from build123d import *

# Parameters (mm, degrees)
F0_R       = 50
F1_DEPTH   = 200
F2_R       = 30
F3_DEPTH   = 150
F1_FACE1_R = 50
F4_R       = 10
F5_DEPTH   = 50
F6_R       = 10
F7_DEPTH   = 150
F8_W       = 25
F8_H       = 25
F8_R       = 10
F9_DEPTH   = 50


# Not quite as in the source:
# - a fillet or chamfer that OpenCascade refuses, or shapes differently, is made with other operations: its cross-section is extruded or revolved along the edge and cut away or added


with BuildPart() as f1:
    # F0 (on Top) → F1 (new body)
    with BuildSketch(Plane.XY):
        Circle(F0_R)
    extrude(amount=F1_DEPTH)

    # F2 (on face) → F3 (cut)
    with BuildSketch(Plane.XY.offset(200)):
        Circle(F2_R)
    extrude(amount=-F3_DEPTH, mode=Mode.SUBTRACT)

    # F1_face1 (on face) + F4 (on face) → F5 (join)
    with BuildSketch(Plane(origin=(0, 0, 0), x_dir=(1, 0, 0), z_dir=(0, 0, -1))):
        Circle(F1_FACE1_R)
    with BuildSketch(Plane(origin=(0, 0, 0), x_dir=(1, 0, 0), z_dir=(0, 0, -1))):
        Circle(F4_R)
    extrude(amount=F5_DEPTH)

    # F6 (on face) → F7 (cut)
    with BuildSketch(Plane(origin=(0, 0, -50), x_dir=(1, 0, 0), z_dir=(0, 0, -1))):
        Circle(F6_R)
    extrude(amount=-F7_DEPTH, mode=Mode.SUBTRACT)

    # F8 (on face) → F9 (join)
    with BuildSketch(Plane.XY.offset(50)):
        Rectangle(F8_W, F8_H)
        Circle(F8_R, mode=Mode.SUBTRACT)
    extrude(amount=F9_DEPTH)

    # F10: chamfer of 15 on 1 edges, made by hand

    # F10_s1 → F10_t2 (revolve)
    with BuildSketch(Plane.XZ):
        Polygon((30, 65), (15, 50), (30, 50), align=None)
    revolve(axis=Axis((0, 0, 50), (0, 0, 1)))


solid = f1.part
Source: CAD feature listing. Evaluate the final solid. Frame: model axes, mm. A direction names the side the tool comes from. Give positions to 0.01 mm unless a question says otherwise; leave off trailing zeros. Write each loop counter-clockwise with the first axis right and the second up, starting at its lowest first coordinate (ties: lowest second). Pieces come first, ordered by that corner, then holes. Notation, with made-up numbers: (40, 64) -> (48, 64) arc R13 cw to (48, 83) -> close; hole circle Ø1 at (81.5, 78.5). An arc over 180 degrees is marked (long way). Return JSON: item names as keys, results as strings. Group by question number.
1. Section A-A, the plane z = 90.5. Output: boundary loops of the cut face in (x, y).
2. Section D-D, the plane z = 38. Output: boundary loops of the cut face in (x, y).
3. Section B-B, the plane x = 0. Output: boundary loops of the cut face in (y, z), then the cut area to 3 significant figures.
4. Pin query (flat end, axial travel): pin 1 Ø12 at (y, z) = (-20, 123.5) entering from +X; pin 2 Ø0.8 at (x, y) = (13.5, -3.5) entering from +Z; pin 3 Ø12.5 at (x, z) = (0.5, 70) entering from -Y. Return the tip coordinate at first contact, or that it passes through.
5. Mould query, pull axis Y, two halves, no side actions, for faces 3 (the face through (47.69, -15.02, 76.75)), 4 (the face through (-0.7, 10.4, -50)), 5 (the face through (-12.5, 0, 75)). Classes: +Y half, -Y half, draft (parallel to the pull), parting line (faces both ways), or undercut.
6. Material intervals for line 1 (X direction, y = 0, z = 29); line 2 (Y direction, x = 0, z = 129.5), sorted ascending. Write a range as from..to.
7. Access query for faces 1 (the face through (-2.17, -9.76, 23.95)), 2 (the face through (-9, 6, 100)). Directions: +Z, -Z, +X, -X, +Y, -Y. A direction counts if a zero-diameter tool reaches every point of the face in a straight line with its end or side. Return the directions, or none.
Determined:
{
 "1": {"outline": "circle Ø100 at (0, 0); (-12.5, -12.5) -> (12.5, -12.5) -> (12.5, 12.5) -> (-12.5, 12.5) -> close; hole circle Ø60 at (0, 0); hole circle Ø20 at (0, 0)"},
 "2": {"outline": "circle Ø100 at (0, 0); hole circle Ø20 at (0, 0)"},
 "3": {"outline": "(-50, -50) -> (-10, -50) -> (-10, 100) -> (-12.5, 100) -> (-12.5, 50) -> (-15, 50) -> (-30, 65) -> (-30, 200) -> (-50, 200) -> close; (10, -50) -> (50, -50) -> (50, 200) -> (30, 200) -> (30, 65) -> (15, 50) -> (12.5, 50) -> (12.5, 100) -> (10, 100) -> close", "area": "14,500 mm2"},
 "4": {"pin 1": "stops at x = 48", "pin 2": "stops at z = 50", "pin 3": "stops at y = -50"},
 "5": {"face 3": "parting line", "face 4": "draft", "face 5": "undercut"},
 "6": {"line 1": "x = -50..-10, 10..50", "line 2": "y = -50..-30, 30..50"},
 "7": {"face 1": "+Z, -Z", "face 2": "+Z"}
}
